```python
from build123d import *

# Parameters (mm, degrees)
SKETCH_1_W        = 30
SKETCH_1_H        = 30
SKETCH_1_W_2      = 26
SKETCH_1_H_2      = 26
EXTRUDE_1_DEPTH   = 250
EXTRUDE_1_2_DEPTH = 250
EXTRUDE_1_3_DEPTH = 250
EXTRUDE_1_4_DEPTH = 250
SKETCH_2_W        = 310
SKETCH_2_H        = 310
EXTRUDE_2_DEPTH   = 3
SKETCH_5_W        = 25
SKETCH_5_H        = 25
SKETCH_5_W_2      = 22
SKETCH_5_H_2      = 22
EXTRUDE_3_DEPTH   = 900
SKETCH_6_W        = 340
SKETCH_6_H        = 340
SKETCH_6_W_2      = 200
SKETCH_6_H_2      = 200
EXTRUDE_4_DEPTH   = 1.5
SKETCH_7_W        = 200
SKETCH_7_H        = 120
EXTRUDE_5_DEPTH   = 1.5
SKETCH_8_W        = 200
SKETCH_8_H        = 1.5
EXTRUDE_6_DEPTH   = 25
SKETCH_9_W        = 200
SKETCH_9_H        = 1.5
EXTRUDE_7_DEPTH   = 25
SKETCH_11_W       = 200
SKETCH_11_H       = 1.5
EXTRUDE_8_DEPTH   = 25


with BuildPart() as part:
    # Sketch 1 → Extrude 1 (new body)
    with BuildSketch(Plane.XY):
        with Locations((-83.068744212, 102.787427317)):
            Rectangle(SKETCH_1_W, SKETCH_1_H)
        with Locations((-83.068744212, 102.787427317)):
            Rectangle(SKETCH_1_W_2, SKETCH_1_H_2, mode=Mode.SUBTRACT)
    extrude(amount=EXTRUDE_1_DEPTH)



with BuildPart() as body_2:
    # Sketch 1 → Extrude 1 2 (new body)
    with BuildSketch(Plane.XY):
        with Locations((176.931255788, 102.787427317)):
            Rectangle(SKETCH_1_W, SKETCH_1_H)
        with Locations((176.931255788, 102.787427317)):
            Rectangle(SKETCH_1_W_2, SKETCH_1_H_2, mode=Mode.SUBTRACT)
    extrude(amount=EXTRUDE_1_2_DEPTH)


with BuildPart() as body_3:
    # Sketch 1 → Extrude 1 3 (new body)
    with BuildSketch(Plane.XY):
        with Locations((-83.068744212, -157.212572683)):
            Rectangle(SKETCH_1_W, SKETCH_1_H)
        with Locations((-83.068744212, -157.212572683)):
            Rectangle(SKETCH_1_W_2, SKETCH_1_H_2, mode=Mode.SUBTRACT)
    extrude(amount=EXTRUDE_1_3_DEPTH)


with BuildPart() as body_4:
    # Sketch 1 → Extrude 1 4 (new body)
    with BuildSketch(Plane.XY):
        with Locations((176.931255788, -157.212572683)):
            Rectangle(SKETCH_1_W, SKETCH_1_H)
        with Locations((176.931255788, -157.212572683)):
            Rectangle(SKETCH_1_W_2, SKETCH_1_H_2, mode=Mode.SUBTRACT)
    extrude(amount=EXTRUDE_1_4_DEPTH)


with BuildPart() as part_1:
    add(part.part)

    add(body_2.part)  # Extrude 2 merges body 2

    add(body_3.part)  # Extrude 2 merges body 3

    add(body_4.part)  # Extrude 2 merges body 4
    # Sketch 2 → Extrude 2 (add)
    with BuildSketch(Plane.XY.offset(250)):
        with Locations((46.931255788, -27.212572683)):
            Rectangle(SKETCH_2_W, SKETCH_2_H)
    extrude(amount=EXTRUDE_2_DEPTH)

    # Sketch 5 → Extrude 3 (add)
    with BuildSketch(Plane.XY.offset(253)):
        with Locations((-65.568744212, 85.287427317)):
            Rectangle(SKETCH_5_W, SKETCH_5_H)
        with Locations((-65.568744212, 85.287427317)):
            Rectangle(SKETCH_5_W_2, SKETCH_5_H_2, mode=Mode.SUBTRACT)
        with Locations((-65.568744212, -139.712572683)):
            Rectangle(SKETCH_5_W, SKETCH_5_H)
        with Locations((-65.568744212, -139.712572683)):
            Rectangle(SKETCH_5_W_2, SKETCH_5_H_2, mode=Mode.SUBTRACT)
        with Locations((159.431255788, -139.712572683)):
            Rectangle(SKETCH_5_W, SKETCH_5_H)
        with Locations((159.431255788, -139.712572683)):
            Rectangle(SKETCH_5_W_2, SKETCH_5_H_2, mode=Mode.SUBTRACT)
        with Locations((159.431255788, 85.287427317)):
            Rectangle(SKETCH_5_W, SKETCH_5_H)
        with Locations((159.431255788, 85.287427317)):
            Rectangle(SKETCH_5_W_2, SKETCH_5_H_2, mode=Mode.SUBTRACT)
    extrude(amount=EXTRUDE_3_DEPTH)

    # Sketch 6 → Extrude 4 (add)
    with BuildSketch(Plane.XY.offset(1153)):
        with Locations((46.931255788, -27.212572683)):
            Rectangle(SKETCH_6_W, SKETCH_6_H)
        with Locations((46.931255788, -27.212572683)):
            Rectangle(SKETCH_6_W_2, SKETCH_6_H_2, mode=Mode.SUBTRACT)
    extrude(amount=EXTRUDE_4_DEPTH)

    # Sketch 7 → Extrude 5 (add)
    with BuildSketch(Plane.XY.offset(623)):
        with Locations((46.931255788, 132.787427317)):
            Rectangle(SKETCH_7_W, SKETCH_7_H)
        with Locations((46.931255788, -187.212572683)):
            Rectangle(SKETCH_7_W, SKETCH_7_H)
    extrude(amount=EXTRUDE_5_DEPTH)

    # Sketch 8 → Extrude 6 (add, symmetric)
    with BuildSketch(Plane(origin=(0, 0, 1003), x_dir=(-1, 0, 0), z_dir=(0, 0, -1))):
        with Locations((-46.931255788, 73.537427317)):
            Rectangle(SKETCH_8_W, SKETCH_8_H)
        with Locations((-46.931255788, -127.962572683)):
            Rectangle(SKETCH_8_W, SKETCH_8_H)
    extrude(amount=EXTRUDE_6_DEPTH, both=True)

    # Sketch 9 → Extrude 7 (add, symmetric)
    with BuildSketch(Plane(origin=(0, 0, 791), x_dir=(-1, 0, 0), z_dir=(0, 0, -1))):
        with Locations((-46.931255788, 73.537427317)):
            Rectangle(SKETCH_9_W, SKETCH_9_H)
        with Locations((-46.931255788, -127.962572683)):
            Rectangle(SKETCH_9_W, SKETCH_9_H)
    extrude(amount=EXTRUDE_7_DEPTH, both=True)

    # Sketch 11 → Extrude 8 (add, symmetric)
    with BuildSketch(Plane(origin=(0, 0, 553), x_dir=(-1, 0, 0), z_dir=(0, 0, -1))):
        with Locations((-46.931255788, -127.962572683)):
            Rectangle(SKETCH_11_W, SKETCH_11_H)
        with Locations((-46.931255788, 73.537427317)):
            Rectangle(SKETCH_11_W, SKETCH_11_H)
    extrude(amount=EXTRUDE_8_DEPTH, both=True)


solid = part_1.part
```
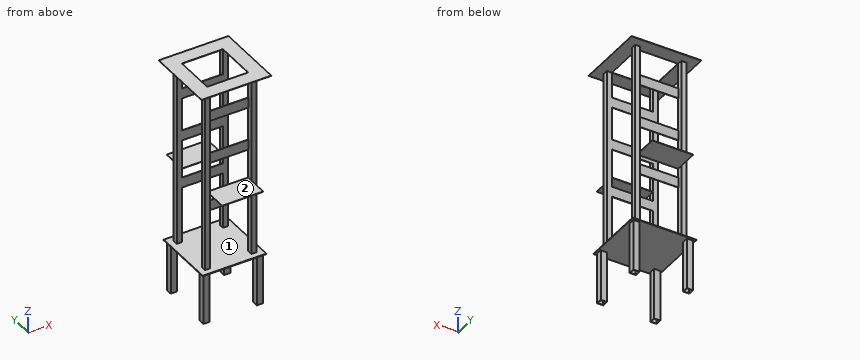
Here's how the part is built. I have some questions about the finished solid (model axes, mm). Face numbers are marked on the shaded views. A direction names the side the tool comes from. Round coordinates to 2 decimals unless told otherwise and drop trailing zeros. Order: outer loops, then holes, each group sorted by start corner. A loop starts at its lowest first (then second) coordinate and runs counter-clockwise, first axis right, second up. Notation, with made-up numbers: (71.5, -35.75) -> (120.5, -35.75) arc R36 ccw to (120.5, 1.25) -> close; hole circle Ø4 at (35, 41.5). An arc over 180 degrees is marked (long way). Use a Markdown table: item, result. Add a question column.
(1) For pin 1 Ø0.8 at (x, y) = (12.5, -128) entering from -Z; pin 2 Ø25 at (x, z) = (29.5, 563) entering from +Y; pin 3 Ø1 at (x, y) = (19.5, -41.5) entering from +Z, each with a flat end and sliding along its axis, tell me the tip position at first contact or that it passes through.
(2) For the marked faces 1 and 2, which set-ups out of +Z, -Z, +X, -X, +Y, -Y let a thin tool reach every point of the face, with its end or its side?
(3) Suppose I cut it at B-B, the plane y = -60. Please give me the cut outline in (x, z), and give its area (3 significant figures).
(4) Suppose I cut it at A-A, the plane z = 429. Count the separate pieces of the cut face and the enclosed holes in it, and give its area (3 significant figures).
(5) I need wall thicknesses on line 1 along Z through (x, y) = (75, -178.5); line 2 along Y through (x, z) = (-90, 215); line 3 along X through (y, z) = (-150.5, 185.5). Which ranges of each line are inside material? Lowest first, please.
Verdict:
| question | item | result |
|---|---|---|
| 1 | pin 1 | z = 250 |
| 1 | pin 2 | y = 74.29 |
| 1 | pin 3 | z = 253 |
| 2 | face 1 | none |
| 2 | face 2 | +Y, -Y |
| 3 | outline | (-123.07, 1153) -> (-53.07, 1153) -> (-53.07, 1154.5) -> (-123.07, 1154.5) -> close; (-108.07, 250) -> (201.93, 250) -> (201.93, 253) -> (-108.07, 253) -> close; (146.93, 1153) -> (216.93, 1153) -> (216.93, 1154.5) -> (146.93, 1154.5) -> close |
| 3 | area | 1,140 mm2 |
| 4 | separate pieces | 4 |
| 4 | enclosed holes | 4 |
| 4 | area | 564 mm2 |
| 5 | line 1 | 250 to 253, 623 to 624.5, 1153 to 1154.5 |
| 5 | line 2 | -172.21 to -170.21, -144.21 to -142.21, 87.79 to 89.79, 115.79 to 117.79 |
| 5 | line 3 | -98.07 to -96.07, -70.07 to -68.07, 161.93 to 163.93, 189.93 to 191.93 |
